Here's how the part is built. I have some questions about the finished solid (model axes, mm). A direction names the side the tool comes from. Give positions to 0.01 mm unless a question says otherwise; leave off trailing zeros. Write each loop counter-clockwise with the first axis right and the second up, starting at its lowest first coordinate (ties: lowest second). Pieces come first, ordered by that corner, then holes. Notation, with made-up numbers: (23, 25) - (50, 25) arc R6 cw to (50, 35) - close; hole circle Ø9 at (24.25, -13). An arc over 180 degrees is marked (long way). Use a Markdown table: item, result.
```python
from build123d import *

# Parameters (mm, degrees)
F1_DEPTH = 28


with BuildPart() as f1:
    # F0 (on Front) → F1 (new body)
    with BuildSketch(Plane.XZ):
        with BuildLine():
            Line((-4.5333905146, 34.6125476062), (-8.0259768292, 34.6125476062))
            Line((-8.0259768292, 34.6125476062), (-8.0259768292, -3.4810174257))
            Line((-8.0259768292, -3.4810174257), (-8.0259768292, -8.127710782))
            add(Edge.make_bspline(
                [(-8.0259768292, -8.127710782), (-4.3456946952, -22.6571589788), (-0.6654125612, -37.1866071756), (8.7871747091, -35.4477465153)],
                knots=[0, 0, 0, 0, 0.4330503534, 0.4330503534, 0.4330503534, 0.4330503534], degree=3))
            Line((8.7871747091, -35.4477465153), (8.7871747091, -30.869955197))
            add(Edge.make_bspline(
                [(-4.5333905146, -3.4810174257), (-0.9766891541, -16.9478294021), (1.169743888, -30.5117774218), (8.7871747091, -30.869955197)],
                knots=[0, 0, 0, 0, 0.5097867068, 0.5097867068, 0.5097867068, 0.5097867068], degree=3))
            Line((-4.5333905146, -3.4810174257), (-4.5333905146, 34.6125476062))
        make_face()
    extrude(amount=F1_DEPTH)


solid = f1.part
```
Item 1: Will these pins go through, and if not, where does the flat tip stop? pin 1 Ø2 at (y, z) = (-18.5, -16) entering from -X; pin 2 Ø6 at (y, z) = (-7.5, 2) entering from +X; pin 3 Ø1.5 at (x, y) = (3.5, -16) entering from -Z.
Values:
| item | result |
|---|---|
| pin 1 | stops at x = -6.25 |
| pin 2 | stops at x = -4.53 |
| pin 3 | stops at z = -34.92 |
Item 2: For faces 1 (the flat face through (-4.533, -14, 15)), 2 (the flat face through (-8.026, -14, 14)), which set-ups out of +Z, -Z, +X, -X, +Y, -Y let a thin tool reach every point of the face, with its end or its side?
Values:
| item | result |
|---|---|
| face 1 | +Z, +X, +Y, -Y |
| face 2 | +Z, -Z, -X, +Y, -Y |
Item 3: If we section it at A-A, the plane z = 10.5: Write out the boundary of the cut face in (x, y), plus the area to 3 significant figures.
Values:
| item | result |
|---|---|
| outline | (-8.03, -28) - (-4.53, -28) - (-4.53, 0) - (-8.03, 0) - close |
| area | 97.8 mm2 |
Item 4: I need wall thicknesses on line 1 along X through (y, z) = (-12.75, 25); line 2 along X through (y, z) = (-19.75, -27.5); line 3 along Z through (x, y) = (1.75, -16.25). Which ranges of each line are inside material? Lowest first, please. Write a range as [from, to].
Values:
| item | result |
|---|---|
| line 1 | x = [-8.03, -4.53] |
| line 2 | x = [-1.97, 3.34] |
| line 3 | z = [-33.13, -24.79] |
